The listing builds one solid part. Answer for the finished solid, in the listing's coordinates (mm). A direction names the side the tool comes from. Coordinates: 2 decimals unless noted, no trailing zeros. Order: outer loops, then holes, each group sorted by start corner. A loop starts at its lowest first (then second) coordinate and runs counter-clockwise, first axis right, second up. Notation, with made-up numbers: (-13, 31.25) -> (7, 31.25) arc R19 ccw to (7, 56.25) -> close; hole circle Ø6 at (-8.5, 49). An arc over 180 degrees is marked (long way). Write each question's results on one line, items separated by ' | '. Start each with the question number.
(1) Straight lines are drawn through the part: L1, parallel to X at y = 6.25, z = 4; L2, parallel to Z at x = -9, y = -3.25; L3, parallel to Y at x = -6.75, z = -1. For each, find the intervals that lie inside material, in ascending order.
(2) Determine the mould class of faces 4 (the face through (8.456, -3.796, 0.167)), 5 (the face through (5.535, -0.867, -3.905)), 6 (the face through (10, 0, 0)) for opening direction X: +X half, -X half, draft (parallel to the pull), parting line (faces both ways), or undercut.
(3) The part is cut by section D-D, the plane x = 1.5. Give the vertices of the cut face in (y, z), then the cut area to 3 significant figures.
(4) A tool of negligible diameter and unlimited length cuts with its end or side. For faces 1 (the face through (3, 3, 3)), 2 (the face through (0.989, -1.172, -8.923)), 3 (the face through (-6.21, -1.08, 4.88)), from which of +Z, -Z, +X, -X, +Y, -Y can it reach the whole face along a straight path? Write none if from no direction.
(5) The part is cut by section C-C, the plane x = -1. Give the vertices of the cut face in (y, z).
(6) Given pin 1 (4 mm diameter, centred on x = -9.5, z = 0, fed in from -Y); pin 2 (10 mm diameter, centred on x = 5, y = 4, fed in from -Z); pin 3 (8 mm diameter, centred on y = -6.5, z = -5, fed in from +X), each flat-ended and moving along its own axis, determine where each tip first touches the part or whether it passes through.
Autodesk Inventor part; units mm, degrees
ref_plane "YZ Plane" through (0, 0, 0) normal (1, 0, 0) x (0, 1, 0)
ref_plane "XZ Plane" through (0, 0, 0) normal (0, 1, 0) x (-1, 0, 0)
ref_plane "XY Plane" through (0, 0, 0) normal (0, 0, 1) x (1, 0, 0)
sketch "Skizze1" plane through (0, 0, 0) normal (0, 0, 1) x (1, 0, 0)
  line L0 (0, 0) -> (0, 4.75)
  line L1 (0, 4.75) -> (3, 4.75)
  line L2 (3, 4.75) -> (3, 4)
  line L3 (3, 4) -> (8, 4)
  line L4 (8, 4) -> (8, 3.8)
  line L5 (8, 3.8) -> (8.9, 3.8)
  line L6 (8.9, 3.8) -> (8.9, 4)
  line L7 (8.9, 4) -> (9.5, 4)
  line L8 (10, 3.5) -> (10, 0)
  line L9 (10, 0) -> (0, 0)
  line L10 (0, 5) -> (-12.25, 5)
  line L11 (-13.5, 3.75) -> (-13.5, 0)
  line L12 (-13.5, 0) -> (0, 0)
  line L13 (9.5, 4) -> (10, 3.5)
  line L14 (-13.5, 3.75) -> (-12.25, 5)
  line L15 (8, 4) -> (8, 0) construction
  line L16 (2, 4.75) -> (2, 9)
  line L17 (2, 9) -> (0, 9)
  line L18 (0, 9) -> (0, 4.75)
  line L19 (3, 4) -> (3, 0) construction
  point P0 (10, 4)
  point P1 (-13.5, 5)
  dimension "d0" = 7.6
  dimension "d1" = 0.5
  dimension "d2" = 0.5
  dimension "d3" = 0.9
  dimension "d4" = 8
  dimension "d5" = 0.6
  dimension "d6" = 9.5
  dimension "d8" = 10
  dimension "d9" = 1.25
  dimension "d10" = 1.25
  dimension "d11" = 13.5
  dimension "d15" = 0
  dimension "d22" = 1
  dimension "d23" = 18
  dimension "d24" = 5
  dimension "d25" = 0
  dimension "d27" = 3
revolve "Umdrehung1" add sketch "Skizze1" angle 360 about axis through (10, 0, 0) along (-1, 0, 0)
thread "Gewinde1"
chamfer "Fase1" distance 0.2 angle 45 3 edges at (3, -4.75, 0) (2, -9, 0) (0, -9, 0)
equation "\"d22\" = JTM_1018_Thickness"
equation "\"d24\" = Bearing_Thickness"
equation "\"Bearing_StepThickness\" = 2"
equation "\"SupportLink_Bearing_StepDia\" = 13"
equation "\"Bearing_Thickness\" = 5"
equation "\"Bearing_Flansch_Thickness\" = 1.1"
equation "\"JTM_1018_Thickness\" = 1"
properties part number "ParallelMech_SupportLink_Distall_JointShaft" material "Edelstahl"
Established:
1) L1: x = 0 to 2 | L2: z = -3.8 to 3.8 | L3: y = -4.9 to 4.9
2) face 4: undercut | face 5: draft | face 6: +X half
3) outline: circle Ø18 at (0, 0) | area: 254 mm^2
4) face 1: +X | face 2: +X, -X | face 3: -X
5) outline: circle Ø10 at (0, 0)
6) pin 1: stops at y = -5 | pin 2: stops at z = -9 | pin 3: stops at x = 3
